from build123d import *

# Parameters (mm, degrees)
SKETCH1_R           = 60
BOSS_EXTRUDE1_DEPTH = 87.5
SKETCH2_R           = 100
BOSS_EXTRUDE2_DEPTH = 10
SKETCH3_R           = 12.5
BOSS_EXTRUDE3_DEPTH = 20


with BuildPart() as part:
    # Sketch1 → Boss-Extrude1 (new, symmetric)
    with BuildSketch(Plane.XY):
        Circle(SKETCH1_R)
    extrude(amount=BOSS_EXTRUDE1_DEPTH, both=True)

    # Sketch2 → Boss-Extrude2 (add)
    with BuildSketch(Plane.XY.offset(87.5)):
        Circle(SKETCH2_R)
        with BuildLine():
            Line((7.5, 80), (7.5, 20))
            ThreePointArc((7.5, 20), (0, 12.5), (-7.5, 20))
            Line((-7.5, 20), (-7.5, 80))
            ThreePointArc((-7.5, 80), (0, 87.5), (7.5, 80))
        make_face(mode=Mode.SUBTRACT)
        with BuildLine():
            Line((80, 7.5), (20, 7.5))
            ThreePointArc((20, 7.5), (12.5, 0), (20, -7.5))
            Line((20, -7.5), (80, -7.5))
            ThreePointArc((80, -7.5), (87.5, 0), (80, 7.5))
        make_face(mode=Mode.SUBTRACT)
        with BuildLine():
            Line((7.5, -80), (7.5, -20))
            ThreePointArc((7.5, -20), (0, -12.5), (-7.5, -20))
            Line((-7.5, -20), (-7.5, -80))
            ThreePointArc((-7.5, -80), (0, -87.5), (7.5, -80))
        make_face(mode=Mode.SUBTRACT)
        with BuildLine():
            Line((-80, -7.5), (-20, -7.5))
            ThreePointArc((-20, -7.5), (-12.5, 0), (-20, 7.5))
            Line((-20, 7.5), (-80, 7.5))
            ThreePointArc((-80, 7.5), (-87.5, 0), (-80, -7.5))
        make_face(mode=Mode.SUBTRACT)
    boss_extrude2 = extrude(amount=BOSS_EXTRUDE2_DEPTH)

    # Sketch3 → Boss-Extrude3 (add)
    with BuildSketch(Plane.XY.offset(97.5)):
        with Locations(Location((0, 0, 0), (0, 0, 179.999859654))):
            Circle(SKETCH3_R)
    boss_extrude3 = extrude(amount=BOSS_EXTRUDE3_DEPTH)

    # Mirror1: Boss-Extrude2 across plane
    add(boss_extrude2.mirror(Plane.XY))

    # Mirror2: Boss-Extrude3 across plane
    add(boss_extrude3.mirror(Plane.XY))


solid = part.part
The model under review builds one solid part; all positions refer to its coordinate system, in mm. A direction names the side the tool comes from. Coordinates: 2 decimals unless noted, no trailing zeros. Loops run counter-clockwise (first coordinate to the right, second up) from the corner with the lowest first, then second, coordinate; pieces in that order, holes last. Notation, with made-up numbers: M -13,75.25 L 31,75.25 A22 cw 31,96.25 Z; hole C -18,-28 d8. An arc over 180 degrees is marked long. Put each result on its own line as item: value. Start each with the question number.
Q1. Add section D-D (z = -10). Write out the cut boundary in (x, y), and give its area (3 significant figures).
Q2. Wall thickness on line 1 (Z direction, x = 6.5, y = 89.5); line 2 (Z direction, x = -27, y = 51); line 3 (X direction, y = 58, z = -96): over which ranges is each line inside the solid? List them lowest first.
Q3. The part is to be moulded in two halves that separate along X. For faces 6 (the flat face through (0, 0, -117.5)), 7 (the cylindrical face through (-0.16, -87.5, -92.43)), say which applies: +X half, -X half, draft (parallel to the pull), parting line (faces both ways), or undercut.
Q4. For faces 1 (the cylindrical face through (0.16, -12.5, 92.43)), 2 (the flat face through (43, -43, -87.5)), 3 (the cylindrical face through (87.5, -0.16, 92.43)), 4 (the cylindrical face through (0.16, -12.5, -92.43)), 5 (the flat face through (0, 0, 117.5)), list the 3-axis set-ups (+Z, -Z, +X, -X, +Y, -Y) from which the entire face can be reached by the end or side of a thin tool; tool diameter is ignored.
Q5. Add section C-C (x = 35.5). Write out the cut boundary in (y, z).
Q6. Clearance check with flat-ended pins moving along their axes: pin 1 (8 mm diameter, centred on y = 30.5, z = 65, fed in from +X); pin 2 (5 mm diameter, centred on x = -34, y = -23, fed in from -Z); pin 3 (4.5 mm diameter, centred on x = 3.5, y = -40, fed in from +Z). State where each tip first meets the part, or that it passes through.
Q7. Add section A-A (y = -51.5). Write out the cut boundary in (x, z), and give its area (3 significant figures).
Q8. Add section B-B (x = -71). Write out the cut boundary in (y, z).
Answers:
1. outline: C 0,0 d120
1. area: 11,300 mm^2
2. line 1: z = -97.5 to -87.5, 87.5 to 97.5
2. line 2: z = -97.5 to 97.5
2. line 3: x = -81.46 to -7.5, 7.5 to 81.46
3. face 6: draft
3. face 7: undercut
4. face 1: +Z
4. face 2: none
4. face 3: +Z, -Z
4. face 4: -Z
4. face 5: +Z, +X, -X, +Y, -Y
5. outline: M -93.49,-97.5 L -7.5,-97.5 L -7.5,-87.5 L 7.5,-87.5 L 7.5,-97.5 L 93.49,-97.5 L 93.49,-87.5 L 48.37,-87.5 L 48.37,87.5 L 93.49,87.5 L 93.49,97.5 L 7.5,97.5 L 7.5,87.5 L -7.5,87.5 L -7.5,97.5 L -93.49,97.5 L -93.49,87.5 L -48.37,87.5 L -48.37,-87.5 L -93.49,-87.5 Z
6. pin 1: stops at x = 53.83
6. pin 2: stops at z = -97.5
6. pin 3: stops at z = 87.5
7. outline: M -85.72,-97.5 L -7.5,-97.5 L -7.5,-87.5 L 7.5,-87.5 L 7.5,-97.5 L 85.72,-97.5 L 85.72,-87.5 L 30.79,-87.5 L 30.79,87.5 L 85.72,87.5 L 85.72,97.5 L 7.5,97.5 L 7.5,87.5 L -7.5,87.5 L -7.5,97.5 L -85.72,97.5 L -85.72,87.5 L -30.79,87.5 L -30.79,-87.5 L -85.72,-87.5 Z
7. area: 13,900 mm^2
8. outline: M -70.42,-97.5 L -7.5,-97.5 L -7.5,-87.5 L -70.42,-87.5 Z; M -70.42,87.5 L -7.5,87.5 L -7.5,97.5 L -70.42,97.5 Z; M 7.5,-97.5 L 70.42,-97.5 L 70.42,-87.5 L 7.5,-87.5 Z; M 7.5,87.5 L 70.42,87.5 L 70.42,97.5 L 7.5,97.5 Z
